Design review of the part built by this model. Coordinates are the model's own, in mm. Face numbers are marked on the shaded views. A direction names the side the tool comes from. Give positions to 0.01 mm unless a question says otherwise; leave off trailing zeros. Write each loop counter-clockwise with the first axis right and the second up, starting at its lowest first coordinate (ties: lowest second). Pieces come first, ordered by that corner, then holes. Notation, with made-up numbers: (-38, 39) -> (1, 39) arc R19 cw to (1, 47) -> close; hole circle Ø6 at (19.5, 34). An arc over 180 degrees is marked (long way). Put each result on its own line as item: value. Start each with the question number.
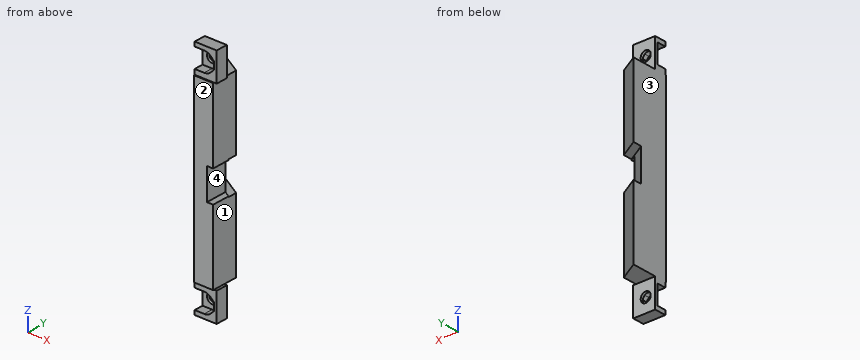
from build123d import *

# Parameters (mm, degrees)
CLAMP_START                      = -20.15
CLAMP_X_COVER_DEPTH              = 37.1
WIRE_START                       = -4.99
WIRE_CHANNEL_X_COVER_Z_5_0_DEPTH = 6.78
WIRE_START_2                     = -4.84
SKETCH3_W                        = 1.6
SKETCH3_H                        = 5.420657937
WIRE_NOTCH_X_COVER_Z_5_0_DEPTH   = 6.48
EAR_START                        = -26.1
SKETCH4_W                        = 4.582851153
SKETCH4_H                        = 2.45
EAR_X_COVER_26_DEPTH             = 5.95
EAR_START_2                      = 16.95
SKETCH5_W                        = 4.582851153
SKETCH5_H                        = 2.45
EAR_X_COVER_17_DEPTH             = 5.95
CUT_EXTRUDE3_START               = 18.7
SKETCH6_R                        = 1.05
CUT_EXTRUDE3_DEPTH               = 2.65
CUT_EXTRUDE4_START               = 18.79
SKETCH7_R                        = 2
CUT_EXTRUDE4_DEPTH               = 1.92
CUT_EXTRUDE5_START               = 18.79
SKETCH8_W                        = 2.082851153
SKETCH8_H                        = 4
CUT_EXTRUDE5_DEPTH               = 1.92
CUT_EXTRUDE6_START               = 18.79
CUT_EXTRUDE6_DEPTH               = 1.92
CUT_EXTRUDE7_START               = 18.79
CUT_EXTRUDE7_DEPTH               = 1.92


with BuildPart() as part:
    # Sketch1 → Clamp +X cover (new body)
    with BuildSketch(Plane.XY.offset(CLAMP_START)):
        Polygon((13.367148847, 18.6), (17.397275866, 18.6), (17.397275866, 24.170102587), (13.367148847, 26.496897507), align=None)
    extrude(amount=CLAMP_X_COVER_DEPTH)

    # Sketch2 → Wire channel +X cover Z -5.0 (cut)
    with BuildSketch(Plane.XY.offset(WIRE_START)):
        Polygon((11.102085338, 27.920102587), (19.762339376, 22.920102587), (18.912339376, 21.447859401), (10.252085338, 26.447859401), align=None)
    extrude(amount=WIRE_CHANNEL_X_COVER_Z_5_0_DEPTH, mode=Mode.SUBTRACT)

    # Sketch3 → Wire notch +X cover Z -5.0 (cut)
    with BuildSketch(Plane.XY.offset(WIRE_START_2)):
        with Locations((16.897275866, 21.210328969)):
            Rectangle(SKETCH3_W, SKETCH3_H)
    extrude(amount=WIRE_NOTCH_X_COVER_Z_5_0_DEPTH, mode=Mode.SUBTRACT)

    # Sketch4 → Ear +X cover -26 (add)
    with BuildSketch(Plane.XY.offset(EAR_START)):
        with Locations((15.658574424, 20.025)):
            Rectangle(SKETCH4_W, SKETCH4_H)
    extrude(amount=EAR_X_COVER_26_DEPTH)

    # Sketch5 → Ear +X cover 17 (add)
    with BuildSketch(Plane.XY.offset(EAR_START_2)):
        with Locations((15.658574424, 20.025)):
            Rectangle(SKETCH5_W, SKETCH5_H)
    extrude(amount=EAR_X_COVER_17_DEPTH)

    # Sketch6 → Cut-Extrude3 (cut)
    with BuildSketch(Plane(origin=(0, 0, 0), x_dir=(1, 0, 0), z_dir=(0, 1, 0)).offset(CUT_EXTRUDE3_START)):
        with Locations(Location((15.35, 23.2, 0), (0, 0, 90))):
            Circle(SKETCH6_R)
        with Locations(Location((15.35, -20, 0), (0, 0, 90))):
            Circle(SKETCH6_R)
    extrude(amount=CUT_EXTRUDE3_DEPTH, mode=Mode.SUBTRACT)

    # Sketch7 → Cut-Extrude4 (cut)
    with BuildSketch(Plane(origin=(0, 0, 0), x_dir=(1, 0, 0), z_dir=(0, 1, 0)).offset(CUT_EXTRUDE4_START)):
        with Locations((15.35, 23.2)):
            Circle(SKETCH7_R)
        with Locations((15.35, -20)):
            Circle(SKETCH7_R)
    extrude(amount=CUT_EXTRUDE4_DEPTH, mode=Mode.SUBTRACT)

    # Sketch8 → Cut-Extrude5 (cut)
    with BuildSketch(Plane(origin=(0, 0, 0), x_dir=(1, 0, 0), z_dir=(0, 1, 0)).offset(CUT_EXTRUDE5_START)):
        with Locations((14.308574424, 23.2)):
            Rectangle(SKETCH8_W, SKETCH8_H)
        with Locations((14.308574424, -20)):
            Rectangle(SKETCH8_W, SKETCH8_H)
    extrude(amount=CUT_EXTRUDE5_DEPTH, mode=Mode.SUBTRACT)

    # Sketch9 → Cut-Extrude6 (cut)
    with BuildSketch(Plane(origin=(0, 0, 0), x_dir=(1, 0, 0), z_dir=(0, 1, 0)).offset(CUT_EXTRUDE6_START)):
        Polygon((15.35, 25.2), (16.764213562, 24.614213562), (17.35, 24.028427125), (17.35, 22.371572875), (16.764213562, 21.785786438), (15.35, 21.2), align=None)
    extrude(amount=CUT_EXTRUDE6_DEPTH, mode=Mode.SUBTRACT)

    # Sketch10 → Cut-Extrude7 (cut)
    with BuildSketch(Plane(origin=(0, 0, 0), x_dir=(1, 0, 0), z_dir=(0, 1, 0)).offset(CUT_EXTRUDE7_START)):
        Polygon((15.35, -18), (16.764213562, -18.585786438), (17.35, -19.171572875), (17.35, -20.828427125), (16.764213562, -21.414213562), (15.35, -22), align=None)
    extrude(amount=CUT_EXTRUDE7_DEPTH, mode=Mode.SUBTRACT)


solid = part.part
Q1. Machinability: for the marked faces 3 and 4, which of the approach directions +Z, -Z, +X, -X, +Y, -Y give a long, thin tool a straight path to every point of the face, cutting with its end or side? Answer none if there is none.
Q2. Take a section at C-C on x = 13.85. Give the boundary of the cut face in (y, z), then the cut area to 3 significant figures.
Q3. Take a section at D-D on z = 8. Give the boundary of the cut face in (x, y).
Q4. Mouldability with a two-part tool opening along Z and no side actions: class the marked faces 1 and 2 as +Z half, -Z half, draft (parallel to the pull), parting line (faces both ways), or undercut.
Q5. Take a section at B-B on y = 19.5. Give the boundary of the cut face in (x, z), then the cut area to 3 significant figures.
Q6. Take a section at A-A on z = -23.2. Give the boundary of the cut face in (x, y).
Q7. To check wall thickness, follow probe 1 along Z at (x, y) = (15.35, 21.1); probe 2 along Z at (x, y) = (17.3, 24); probe 3 along Z at (x, y) = (16.8, 20.25). State the ranges of each line that lie inside material, in increasing order. Write a range as from..to.
Q8. For pin 1 (0.8 mm diameter, centred on y = 20, z = 20, fed in from -X); pin 2 (0.6 mm diameter, centred on x = 18, y = 20, fed in from -Z); pin 3 (1.5 mm diameter, centred on x = 14.5, y = 24.5, fed in from +Z); pin 4 (1.5 mm diameter, centred on y = 25, z = -10, fed in from +X), all flat-tipped, find the tip position at first contact; note any pin that passes through.
Result:
1. face 3: +Z, -Z, -X, +Y, -Y
1. face 4: +X, +Y, -Y
2. outline: (18.6, -20.15) -> (18.8, -20.15) -> (18.8, -21.2) -> (20.71, -21.2) -> (20.71, -25.2) -> (18.8, -25.2) -> (18.8, -26.1) -> (21.25, -26.1) -> (21.25, -20.15) -> (26.22, -20.15) -> (26.22, -4.99) -> (24.37, -4.99) -> (24.37, 1.79) -> (26.22, 1.79) -> (26.22, 16.95) -> (21.25, 16.95) -> (21.25, 22.9) -> (18.8, 22.9) -> (18.8, 22) -> (20.71, 22) -> (20.71, 18) -> (18.8, 18) -> (18.8, 16.95) -> (18.6, 16.95) -> close
2. area: 284 mm^2
3. outline: (13.37, 18.6) -> (17.4, 18.6) -> (17.4, 24.17) -> (13.37, 26.5) -> close
4. face 1: undercut
4. face 2: draft
5. outline: (13.37, -26.1) -> (17.95, -26.1) -> (17.95, -20.15) -> (17.4, -20.15) -> (17.4, -4.84) -> (16.1, -4.84) -> (16.1, 1.64) -> (17.4, 1.64) -> (17.4, 16.95) -> (17.95, 16.95) -> (17.95, 22.9) -> (13.37, 22.9) -> (13.37, 22) -> (15.35, 22) arc R2 cw to (16.76, 21.41) -> (17.35, 20.83) -> (17.35, 19.17) -> (16.76, 18.59) arc R2 cw to (15.35, 18) -> (13.37, 18) -> (13.37, -21.2) -> (15.35, -21.2) arc R2 cw to (16.76, -21.79) -> (17.35, -22.37) -> (17.35, -24.03) -> (16.76, -24.61) arc R2 cw to (15.35, -25.2) -> (13.37, -25.2) -> close
5. area: 167 mm^2
6. outline: (13.37, 20.71) -> (14.3, 20.71) -> (14.3, 21.25) -> (13.37, 21.25) -> close; (16.4, 20.71) -> (17.35, 20.71) -> (17.35, 18.8) -> (17.95, 18.8) -> (17.95, 21.25) -> (16.4, 21.25) -> close
7. probe 1: z = -26.1..-24.25, -22.15..18.95, 21.05..22.9
7. probe 2: z = -20.15..-4.99, 1.79..16.95
7. probe 3: z = -26.1..-24.58, -21.82..-4.84, 1.64..18.62, 21.38..22.9
8. pin 1: stops at x = 17.35
8. pin 2: stops at z = -26.1
8. pin 3: stops at z = 16.95
8. pin 4: stops at x = 17.26
